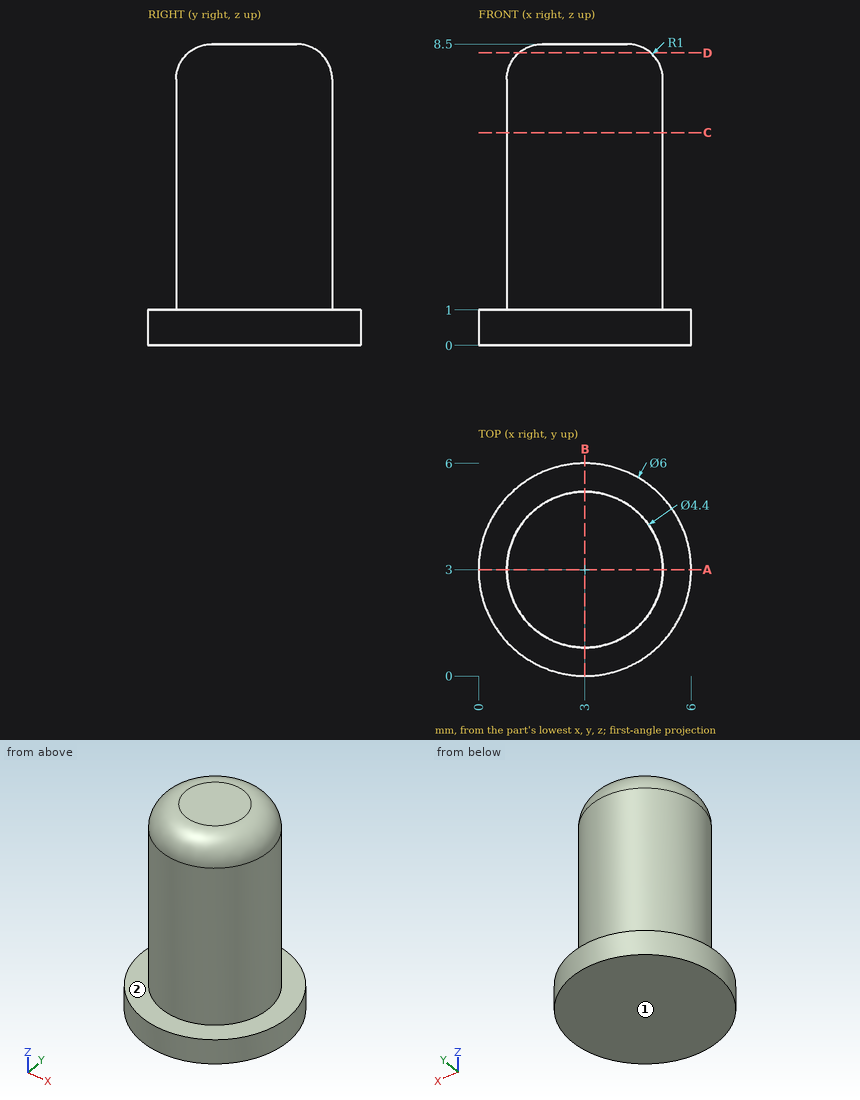
The drawing under review shows one solid part. Ordinate dimensions are in mm from its lowest x, y, z. A direction names the side the tool comes from. Round coordinates to 2 decimals unless told otherwise and drop trailing zeros. Write each loop counter-clockwise with the first axis right and the second up, starting at its lowest first coordinate (ties: lowest second). Pieces come first, ordered by that corner, then holes. Notation, with made-up numbers: (-31.5, 12) - (16.5, 12) arc R8 cw to (16.5, 21) - close; hole circle Ø3 at (63, -21). An arc over 180 degrees is marked (long way). Put each result on its own line as item: value.
Q1. We need section D-D (z = 8.25). Give the boundary of the cut face in (x, y).
Solved:
outline: circle Ø3.72 at (3, 3)
Q2. We need section C-C (z = 6). Give the boundary of the cut face in (x, y).
Solved:
outline: circle Ø4.4 at (3, 3)
Q3. Machinability: for the marked faces 1 and 2, which of the approach directions +Z, -Z, +X, -X, +Y, -Y give a long, thin tool a straight path to every point of the face, cutting with its end or side? Answer none if there is none.
Solved:
face 1: -Z, +X, -X, +Y, -Y
face 2: +Z
Q4. We need section A-A (y = 3). Give the boundary of the cut face in (x, z), and give its area (3 significant figures).
Solved:
outline: (0, 0) - (6, 0) - (6, 1) - (5.2, 1) - (5.2, 7.5) arc R1 ccw to (4.2, 8.5) - (1.8, 8.5) arc R1 ccw to (0.8, 7.5) - (0.8, 1) - (0, 1) - close
area: 38.6 mm2
Q5. Wall thickness on probe 1 along Z at (x, y) = (3.2, 5.75); probe 2 along X at (y, z) = (1.25, 3); probe 3 along Y at (x, z) = (2.5, 3.5): over which ranges is each line inside the solid? List them lowest first.
Solved:
probe 1: z = 0 to 1
probe 2: x = 1.67 to 4.33
probe 3: y = 0.86 to 5.14
Q6. Insertion check: pin 1 Ø1.5 at (x, y) = (5, 1.5) entering from +Z; pin 2 Ø1.5 at (x, z) = (4, 6.5) entering from -Y; pin 3 Ø1.5 at (x, z) = (4, 2) entering from +Y. Each pin has a flat end and moves straight along its axis. Give the tip position at first contact, or say it passes through.
Solved:
pin 1: stops at z = 8.34
pin 2: stops at y = 0.81
pin 3: stops at y = 5.19
